Can you work these out from the model? Positions are in its coordinate system, mm. Give positions to 0.01 mm unless a question says otherwise; leave off trailing zeros. Order: outer loops, then holes, each group sorted by start corner. A loop starts at its lowest first (then second) coordinate and runs counter-clockwise, first axis right, second up. Notation, with made-up numbers: M -24,61.25 L -12,61.25 A25 cw -12,85.25 Z; hole C 88,-27.5 d11. An arc over 180 degrees is marked long. Write each question's results on one line, items separated by ' | '.
from build123d import *

# Parameters (mm, degrees)
CROQUIS1_W              = 2.46
CROQUIS1_H              = 2.46
SALIENTE_EXTRUIR1_DEPTH = 2.37
CROQUIS2_W              = 0.64
CROQUIS2_H              = 0.64
SALIENTE_EXTRUIR2_DEPTH = 6.45
CROQUIS3_W              = 0.64
CROQUIS3_H              = 0.64
SALIENTE_EXTRUIR3_DEPTH = 2
CHAFL_N1_SIZE           = 0.2
CHAFL_N2_SIZE           = 0.2
CHAFL_N3_SIZE           = 0.2
CHAFL_N4_SIZE           = 0.2
CHAFL_N5_SIZE           = 0.1
CHAFL_N6_SIZE           = 0.1
CHAFL_N7_SIZE           = 0.2
CHAFL_N8_SIZE           = 0.2


with BuildPart() as part:
    # Croquis1 → Saliente-Extruir1 (new body)
    with BuildSketch(Plane.XY):
        with Locations((-36.003107302, -31.574436279)):
            Rectangle(CROQUIS1_W, CROQUIS1_H)
    extrude(amount=SALIENTE_EXTRUIR1_DEPTH)

    # Croquis2 → Saliente-Extruir2 (add)
    with BuildSketch(Plane(origin=(0, -30.344436279, 0), x_dir=(1, 0, 0), z_dir=(0, 1, 0))):
        with Locations((-36.003107302, -1.185)):
            Rectangle(CROQUIS2_W, CROQUIS2_H)
    extrude(amount=SALIENTE_EXTRUIR2_DEPTH)

    # Croquis3 → Saliente-Extruir3 (add)
    with BuildSketch(Plane.XZ.offset(32.804436279)):
        with Locations((-36.003107302, 1.185)):
            Rectangle(CROQUIS3_W, CROQUIS3_H)
    extrude(amount=SALIENTE_EXTRUIR3_DEPTH)

    # Chaflán1
    chafl_n1_edges = [part.edges().sort_by_distance(p)[0] for p in [
        (-37.233107302, -31.574436279, 2.37),
    ]]
    chamfer(chafl_n1_edges, length=CHAFL_N1_SIZE)

    # Chaflán2
    chafl_n2_edges = [part.edges().sort_by_distance(p)[0] for p in [
        (-34.773107302, -31.574436279, 2.37),
    ]]
    chamfer(chafl_n2_edges, length=CHAFL_N2_SIZE)

    # Chaflán3
    chafl_n3_edges = [part.edges().sort_by_distance(p)[0] for p in [
        (-34.773107302, -31.574436279, 0),
    ]]
    chamfer(chafl_n3_edges, length=CHAFL_N3_SIZE)

    # Chaflán4
    chafl_n4_edges = [part.edges().sort_by_distance(p)[0] for p in [
        (-37.233107302, -31.574436279, 0),
    ]]
    chamfer(chafl_n4_edges, length=CHAFL_N4_SIZE)

    # Chaflán5
    chafl_n5_edges = [part.edges().sort_by_distance(p)[0] for p in [
        (-35.683107302, -23.894436279, 1.185),
    ]]
    chamfer(chafl_n5_edges, length=CHAFL_N5_SIZE)

    # Chaflán6
    chafl_n6_edges = [part.edges().sort_by_distance(p)[0] for p in [
        (-36.323107302, -23.894436279, 1.185),
    ]]
    chamfer(chafl_n6_edges, length=CHAFL_N6_SIZE)

    # Chaflán7
    chafl_n7_edges = [part.edges().sort_by_distance(p)[0] for p in [
        (-35.683107302, -34.804436279, 1.185),
    ]]
    chamfer(chafl_n7_edges, length=CHAFL_N7_SIZE)

    # Chaflán8
    chafl_n8_edges = [part.edges().sort_by_distance(p)[0] for p in [
        (-36.323107302, -34.804436279, 1.185),
    ]]
    chamfer(chafl_n8_edges, length=CHAFL_N8_SIZE)


solid = part.part
(1) I need wall thicknesses on L1, parallel to Y at x = -35.3, z = 0.85; L2, parallel to X at y = -26, z = 1.25; L3, parallel to Z at x = -35.8, y = -25 (3 decimals). Which ranges of each line are inside material? Lowest first, please. Write a range as from..to.
Data:
L1: y = -32.8..-30.34 | L2: x = -36.32..-35.68 | L3: z = 0.865..1.505
(2) Imagine slicing it at C-C, the plane x = -36.9. Write out the boundary of the cut face in (y, z).
Data:
outline: M -32.8,0 L -30.34,0 L -30.34,2.37 L -32.8,2.37 Z
(3) Imagine slicing it at A-A, the plane z = 1.1. Write out the boundary of the cut face in (x, y), plus the area to 3 significant figures.
Data:
outline: M -37.23,-32.8 L -36.32,-32.8 L -36.32,-34.6 L -36.12,-34.8 L -35.88,-34.8 L -35.68,-34.6 L -35.68,-32.8 L -34.77,-32.8 L -34.77,-30.34 L -35.68,-30.34 L -35.68,-23.99 L -35.78,-23.89 L -36.22,-23.89 L -36.32,-23.99 L -36.32,-30.34 L -37.23,-30.34 Z | area: 11.4 mm2
(4) Will these pins go through, and if not, where does the flat tip stop? P1, Ø1.2, axis at x = -35.5, z = 1.5, coming from the -Y side; P2, Ø0.7, axis at y = -27.5, z = 1, coming from the +X side; P3, Ø1, axis at y = -25.5, z = 1, coming from the -X side; P4, Ø0.7, axis at x = -36, y = -34, coming from the -Z side (3 decimals).
Data:
P1: stops at y = -34.8 | P2: stops at x = -35.68 | P3: stops at x = -36.32 | P4: stops at z = 0.865
(5) Imagine slicing it at B-B, the plane y = -28.5. Write out the boundary of the cut face in (x, z) (3 decimals), plus the area to 3 significant figures.
Data:
outline: M -36.323,0.865 L -35.683,0.865 L -35.683,1.505 L -36.323,1.505 Z | area: 0.410 mm2
